Design review of the part built by this model. Coordinates are the model's own, in mm. Coordinates: 2 decimals unless noted, no trailing zeros. Order: outer loops, then holes, each group sorted by start corner. A loop starts at its lowest first (then second) coordinate and runs counter-clockwise, first axis right, second up. Notation, with made-up numbers: (54, -30.5) -> (110, -30.5) arc R21 cw to (110, -0.5) -> close; hole circle Ø5 at (61, 77). An arc over 180 degrees is marked (long way). Use a Markdown table: item, result. Add a question column.
Q1. Wall thickness on probe 1 along Y at (x, z) = (0, 2.75); probe 2 along Y at (x, z) = (-51, 4.5); probe 3 along Y at (x, z) = (-22, 3.5): over which ranges is each line inside the solid? List them lowest first.
Q2. Add section C-C (z = 4.75). Count the separate pieces of the cut face and the enclosed holes in it, then the cut area to 3 significant figures.
Q3. Add section D-D (y = 106). State the section outline as (x, z) points, then the cut area to 3 significant figures.
Q4. Insertion check: pin 1 (2 mm diameter, centred on x = 26, z = 1.5, fed in from +Y); pin 2 (3 mm diameter, centred on x = 3.91, y = 286.91, fed in from +Z); pin 3 (7 mm diameter, centred on x = -51, y = 57, fed in from +Z); pin 4 (1 mm diameter, centred on x = -30, z = 4.5, fed in from +Y). Each pin has a flat end and moves straight along its axis. Give the tip position at first contact, or say it passes through.
Q5. Add section A-A (y = 216). State the section outline as (x, z) points.
Q6. Add section B-B (x = 43.5). State the section outline as (y, z) points, then the cut area to 4 significant figures.
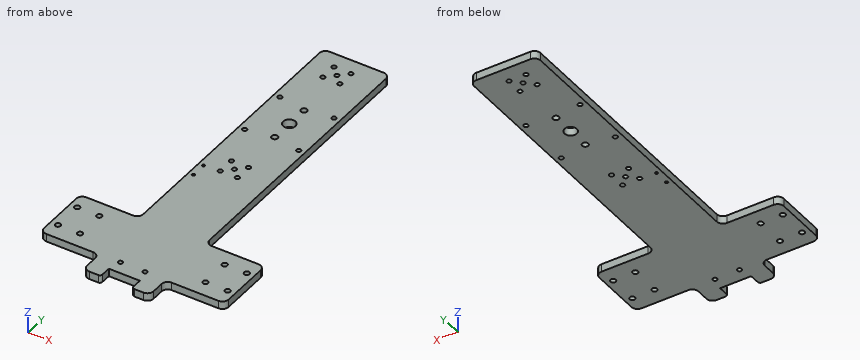
from build123d import *

# Parameters (mm, degrees)
BOSS_EXTRUDE1_DEPTH           = 6.35
FILLET1_R                     = 5
SKETCH3_R                     = 5
CUT_EXTRUDE1_DEPTH            = 7.35
F_6_CLEARANCE_HOLE1_D         = 3.6576
CUT_EXTRUDE2_DEPTH            = 7.35
F_10_CLEARANCE_HOLE2_D        = 4.9784
F_6_CLEARANCE_HOLE2_D         = 3.6576
F_8_CLEARANCE_HOLE1_D         = 4.3053
TAP_DRILL_FOR_4_40_TAP1_D     = 2.2606
TAP_DRILL_FOR_4_40_TAP1_DEPTH = 6.35
TAP_DRILL_FOR_4_40_TAP1_TIP   = 0.679152758
FILLET2_R                     = 2


with BuildPart() as part:
    # Sketch1 → Boss-Extrude1 (new body)
    with BuildSketch(Plane.XY):
        Polygon((-27, 70), (-27, 300), (27, 300), (27, 70), (75, 70), (75, 20), (27, 20), (27, 0), (-27, 0), (-27, 20), (-75, 20), (-75, 70), align=None)
    extrude(amount=BOSS_EXTRUDE1_DEPTH)

    # Fillet1
    fillet1_edges = [part.edges().sort_by_distance(p)[0] for p in [
        (-75, 70, 3.175),
        (-27, 70, 3.175),
        (-27, 300, 3.175),
        (27, 300, 3.175),
        (27, 70, 3.175),
        (75, 70, 3.175),
        (75, 20, 3.175),
        (27, 20, 3.175),
        (27, 0, 3.175),
        (-27, 0, 3.175),
        (-27, 20, 3.175),
        (-75, 20, 3.175),
    ]]
    fillet(fillet1_edges, radius=FILLET1_R)

    # Sketch3 → Cut-Extrude1 (cut, through all)
    with BuildSketch(Plane.XY.offset(6.35)):
        with Locations((0, 216)):
            Circle(SKETCH3_R)
    extrude(amount=-CUT_EXTRUDE1_DEPTH, mode=Mode.SUBTRACT)

    # #6 Clearance Hole1 (through all)
    with Locations(Plane.XY.offset(6.35)):
        with Locations((-22, 238), (-22, 194), (22, 194), (22, 238), (-9.914797213, 273.085202787), (-9.914797213, 286.914797213), (3.914797213, 286.914797213), (3.914797213, 273.085202787), (-9.914797213, 158.914797213), (3.914797213, 158.914797213), (3.914797213, 145.085202787), (-9.914797213, 145.085202787), (-3, 280), (-3, 152)):
            Hole(F_6_CLEARANCE_HOLE1_D / 2)

    # Sketch6 → Cut-Extrude2 (cut, through all)
    with BuildSketch(Plane.XY.offset(6.35)):
        Polygon((-12.7, 0), (-12.6, 10), (12.6, 10), (12.7, 0), align=None)
    extrude(amount=-CUT_EXTRUDE2_DEPTH, mode=Mode.SUBTRACT)

    # #10 Clearance Hole2 (through all)
    with Locations(Plane.XY.offset(6.35)):
        with Locations((0, 197.75), (0, 234.25)):
            Hole(F_10_CLEARANCE_HOLE2_D / 2)

    # #6 Clearance Hole2 (through all)
    with Locations(Plane(origin=(-10, 20.4648, 6.35), x_dir=(1, 0, 0), z_dir=(0, 0, 1))):
        with Locations((0, 0), (20, 0)):
            Hole(F_6_CLEARANCE_HOLE2_D / 2)

    # #8 Clearance Hole1 (through all)
    with Locations(Plane(origin=(51, 57, 6.35), x_dir=(1, 0, 0), z_dir=(0, 0, 1))):
        with Locations((0, 0), (18, 0), (18, -24), (0, -24), (-102, 0), (-120, 0), (-120, -24), (-102, -24)):
            Hole(F_8_CLEARANCE_HOLE1_D / 2)

    # Tap Drill for #4-40 Tap1
    with Locations(Plane(origin=(-23, 131.426, 6.35), x_dir=(1, 0, 0), z_dir=(0, 0, 1))):
        with Locations((0, 0), (0, 12.7)):
            Hole(TAP_DRILL_FOR_4_40_TAP1_D / 2, depth=TAP_DRILL_FOR_4_40_TAP1_DEPTH)
            with Locations((0, 0, -(TAP_DRILL_FOR_4_40_TAP1_DEPTH + TAP_DRILL_FOR_4_40_TAP1_TIP / 2))):  # 118° drill point
                Cone(0, TAP_DRILL_FOR_4_40_TAP1_D / 2, TAP_DRILL_FOR_4_40_TAP1_TIP, mode=Mode.SUBTRACT)

    # Fillet2
    fillet2_edges = [part.edges().sort_by_distance(p)[0] for p in [
        (12.7, 0, 3.175),
        (-12.7, 0, 3.175),
    ]]
    fillet(fillet2_edges, radius=FILLET2_R)


solid = part.part
Established:
| question | item | result |
|---|---|---|
| 1 | probe 1 | 10 to 195.26, 200.24 to 211, 221 to 231.76, 236.74 to 300 |
| 1 | probe 2 | 20 to 30.85, 35.15 to 54.85, 59.15 to 70 |
| 1 | probe 3 | 0 to 130.9, 131.95 to 143.6, 144.65 to 192.17, 195.83 to 236.17, 239.83 to 300 |
| 2 | separate pieces | 1 |
| 2 | enclosed holes | 29 |
| 2 | area | 20,300 mm^2 |
| 3 | outline | (-27, 0) -> (27, 0) -> (27, 6.35) -> (-27, 6.35) -> close |
| 3 | area | 343 mm^2 |
| 4 | pin 1 | y = 299 |
| 4 | pin 2 | through |
| 4 | pin 3 | z = 6.35 |
| 4 | pin 4 | y = 70.67 |
| 5 | outline | (-27, 0) -> (-5, 0) -> (-5, 6.35) -> (-27, 6.35) -> close; (5, 0) -> (27, 0) -> (27, 6.35) -> (5, 6.35) -> close |
| 6 | outline | (20, 0) -> (70, 0) -> (70, 6.35) -> (20, 6.35) -> close |
| 6 | area | 317.5 mm^2 |
